Geometry check sheet. Reference: the model listing, model coordinates, mm. Give positions to 0.01 mm unless a question says otherwise; leave off trailing zeros. Loops run counter-clockwise (first coordinate to the right, second up) from the corner with the lowest first, then second, coordinate; pieces in that order, holes last.
```python
from build123d import *

# Parameters (mm, degrees)
SKETCH1_R            = 2
BOSS_EXTRUDE1_DEPTH  = 1.5875
FILLET2_R            = 1.778
M4_CLEARANCE_HOLE2_D = 4.5


with BuildPart() as part:
    # Sketch1 → Boss-Extrude1 (new body)
    with BuildSketch(Plane.XY):
        with BuildLine():
            Line((-3.078924099, -28.617866551), (2.159951047, -28.617866551))
            Line((2.159951047, -28.617866551), (7.399260817, -28.617866551))
            Line((7.399260817, -28.617866551), (7.399260817, 14.567438128))
            Line((7.399260817, 14.567438128), (7.399260817, 29.567438098))
            Line((7.399260817, 29.567438098), (13.897648784, 51.719401208))
            ThreePointArc((13.897648784, 51.719401208), (2.158996515, 44.568125735), (-9.579655755, 51.719401208))
            Line((-9.579655755, 51.719401208), (-3.078924099, 29.568125765))
            Line((-3.078924099, 29.568125765), (-3.078924099, -28.617866551))
        make_face()
        with BuildLine():
            ThreePointArc((4.159951047, -14.006866551), (3.574164609, -15.421080114), (2.159951047, -16.006866551))
            ThreePointArc((2.159951047, -16.006866551), (0.745737485, -12.592652989), (4.159951047, -14.006866551))
        make_face(mode=Mode.SUBTRACT)
        with Locations((2.159951047, 14.957125769)):
            Circle(SKETCH1_R, mode=Mode.SUBTRACT)
    extrude(amount=BOSS_EXTRUDE1_DEPTH)

    # Fillet2
    fillet2_edges = [part.edges().sort_by_distance(p)[0] for p in [
        (-9.579655755, 51.719401208, 0.79375),
        (13.897648784, 51.719401208, 0.79375),
        (7.399260817, -28.617866551, 0.79375),
        (-3.078924099, -28.617866551, 0.79375),
    ]]
    fillet(fillet2_edges, radius=FILLET2_R)

    # M4 Clearance Hole2 (through all)
    with Locations(Plane.XY.offset(1.5875)):
        with Locations((2.159951047, 14.957125769), (2.159951047, -14.006866551)):
            Hole(M4_CLEARANCE_HOLE2_D / 2)


solid = part.part
```
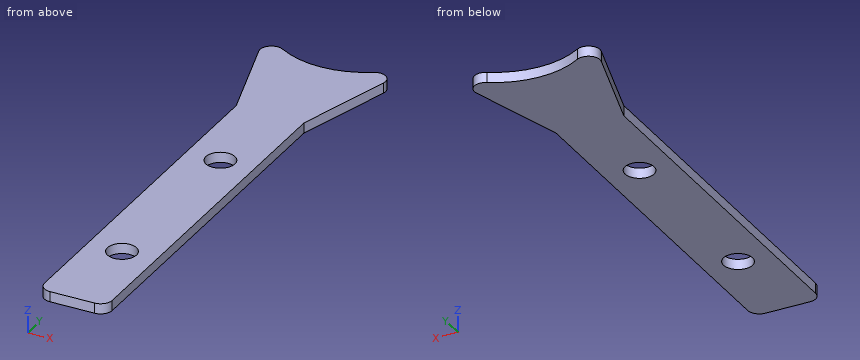
1) Scan lines: line 1 along Y through (x, z) = (3.25, 1.5); line 2 along X through (y, z) = (-8, 1); line 3 along X through (y, z) = (-12, 1.1). Record each from-to range of solid material in increasing order.
2) Sectioned sample at A-A on y = -15. Enter the section's corners in (x, z), plus the area to 3 significant figures.
3) Sectioned sample at B-B on x = 2.5. Enter the section's corners in (y, z), plus the area to 3 significant figures.
4) Depth check by flat-ended pin: P1, Ø2.5, axis at x = 2.16, y = -14.01, coming from the +Z side; P2, Ø3, axis at x = -1.5, y = 8.5, coming from the -Z side; P3, Ø0.5, axis at y = -4.5, z = 0.5, coming from the -X side. Enter the tip coordinate at first touch or a pass-through.
5) Sectioned sample at C-C on z = 0.4. Enter the section's corners in (x, y).
6) Sectioned sample at D-D on y = 6.5. Enter the section's corners in (x, z), plus the area to 3 significant figures.
Determined:
1. line 1: y = -28.62 to -15.98, -12.04 to 12.99, 16.93 to 44.61
1. line 2: x = -3.08 to 7.4
1. line 3: x = -3.08 to 1.14, 3.18 to 7.4
2. outline: (-3.08, 0) - (0.14, 0) - (0.14, 1.59) - (-3.08, 1.59) - close; (4.18, 0) - (7.4, 0) - (7.4, 1.59) - (4.18, 1.59) - close
2. area: 10.2 mm2
3. outline: (-28.62, 0) - (-16.23, 0) - (-16.23, 1.59) - (-28.62, 1.59) - close; (-11.78, 0) - (12.73, 0) - (12.73, 1.59) - (-11.78, 1.59) - close; (17.18, 0) - (44.57, 0) - (44.57, 1.59) - (17.18, 1.59) - close
3. area: 102 mm2
4. P1: passes through
4. P2: stops at z = 0
4. P3: stops at x = -3.08
5. outline: (-7.48, 44.56) - (-3.08, 29.57) - (-3.08, -26.84) arc R1.78 ccw to (-1.3, -28.62) - (5.62, -28.62) arc R1.78 ccw to (7.4, -26.84) - (7.4, 29.57) - (11.8, 44.56) arc R1.78 ccw to (9.15, 46.57) arc R13.21 cw to (-4.83, 46.57) arc R1.78 ccw to start; hole circle Ø4.5 at (2.16, -14.01); hole circle Ø4.5 at (2.16, 14.96)
6. outline: (-3.08, 0) - (7.4, 0) - (7.4, 1.59) - (-3.08, 1.59) - close
6. area: 16.6 mm2
